from build123d import *

# Parameters (mm, degrees)
F0_W            = 50
F0_H            = 25
F0_R            = 1.6
F0_R_2          = 3.15
F1_DEPTH        = 2.5
F2_R            = 1.5
F3_DEPTH        = 25
F3_COPIES_COUNT = 3
F4_W            = 1.5
F4_H            = 21
F5_DEPTH        = 2


# Not quite as in the source:
# - a pattern or mirror of a feature is missing from the dataset's text; its kind, count and spacing are read off the source's solid


with BuildPart() as f1:
    # F0 (on Top) → F1 (new body)
    with BuildSketch(Plane.XY):
        Rectangle(F0_W, F0_H)
        with Locations((-20, 0)):
            Circle(F0_R, mode=Mode.SUBTRACT)
        Circle(F0_R_2, mode=Mode.SUBTRACT)
        with Locations((20, 0)):
            Circle(F0_R, mode=Mode.SUBTRACT)
    extrude(amount=F1_DEPTH)

    # F2 (on face) → F3 (cut)
    with BuildSketch(Plane.XY.offset(2.5)):
        with Locations((0, 8)):
            Circle(F2_R)
    f3 = extrude(amount=-F3_DEPTH, mode=Mode.SUBTRACT)

    # F3_copies: F3 ×3 about axis
    f3_copies_axis = Axis((0, 0, 0), (0, 0, 1))
    for i in range(1, F3_COPIES_COUNT):
        add(f3.rotate(f3_copies_axis, i * 360 / F3_COPIES_COUNT), mode=Mode.SUBTRACT)

    # F4 (on face) → F5 (join)
    with BuildSketch(Plane.XY.offset(2.5)):
        Polygon((25, 12.5), (-25, 12.5), (-25, 10.5), (-5, 10.5), (-3.5, 10.5), (3.5, 10.5), (5, 10.5), (25, 10.5), align=None)
        with Locations((-4.25, 0)):
            Rectangle(F4_W, F4_H)
        with Locations((4.25, 0)):
            Rectangle(F4_W, F4_H)
        Polygon((-3.5, -10.5), (-5, -10.5), (-25, -10.5), (-25, -12.5), (25, -12.5), (25, -10.5), (5, -10.5), (3.5, -10.5), align=None)
    extrude(amount=F5_DEPTH)


solid = f1.part
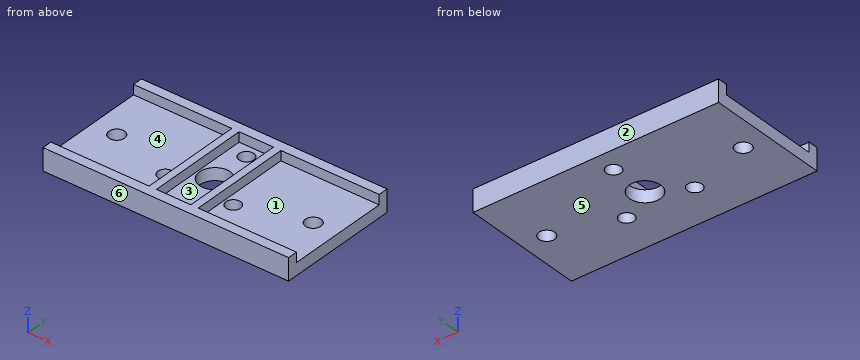
Here's how the part is built. I have some questions about the finished solid (model axes, mm). Face numbers are marked on the shaded views. A direction names the side the tool comes from. Give positions to 0.01 mm unless a question says otherwise; leave off trailing zeros. Loops run counter-clockwise (first coordinate to the right, second up) from the corner with the lowest first, then second, coordinate; pieces in that order, holes last. Notation, with made-up numbers: (-21, 30) -> (-10, 30) arc R31 cw to (-10, 66) -> close; hole circle Ø2 at (28, 68.25). An arc over 180 degrees is marked (long way). Answer as a JSON object with one key per item and string values. Group by question number.
Item 1: Will these pins go through, and if not, where does the flat tip stop? pin 1 (1.9 mm diameter, centred on x = -20, y = 0, fed in from -Z); pin 2 (2 mm diameter, centred on y = 0, z = 4, fed in from -X); pin 3 (2 mm diameter, centred on y = -2, z = 4, fed in from +X); pin 4 (6 mm diameter, centred on x = 8.5, y = -5, fed in from +Z).
Item 2: Imagine slicing it at A-A on y = 0. Write out the boundary of the cut face in (x, z).
Item 3: I need wall thicknesses on L1, parallel to Y at x = 0, z = 1.9; L2, parallel to Y at x = -20, z = 1.35; L3, parallel to X at y = -8, z = 3.45. Which ranges of each line are inside material? Lowest first, please.
Item 4: Imagine slicing it at B-B on x = -20. Write out the boundary of the cut face in (y, z).
Item 5: Imagine slicing it at C-C on x = 0. Write out the boundary of the cut face in (y, z).
Item 6: Imagine slicing it at D-D on y = -4. Write out the boundary of the cut face in (x, z), then the cut area to 3 significant figures.
Item 7: Thinking about a two-plate mould opening in Y: for the marked faces 4, 5 and 6, which applies, pulls with the +Y half, pulls with the -Y half, needs draft (parallel to the pull), parting line crosses it, or undercut?
Item 8: On a 3-axis mill with a long thin cutter (end or side, diameter ignored), from which of +Z, -Z, +X, -X, +Y, -Y can I reach the whole of each face in a straight line? I mean the marked faces 1, 2 and 3. Say none if no direction works.
Answer list:
{
 "1": {"pin 1": "passes through", "pin 2": "stops at x = -5", "pin 3": "stops at x = 5", "pin 4": "stops at z = 2.5"},
 "2": {"outline": "(-25, 0) -> (-21.6, 0) -> (-21.6, 2.5) -> (-25, 2.5) -> close; (-18.4, 0) -> (-3.15, 0) -> (-3.15, 2.5) -> (-3.5, 2.5) -> (-3.5, 4.5) -> (-5, 4.5) -> (-5, 2.5) -> (-18.4, 2.5) -> close; (3.15, 0) -> (18.4, 0) -> (18.4, 2.5) -> (5, 2.5) -> (5, 4.5) -> (3.5, 4.5) -> (3.5, 2.5) -> (3.15, 2.5) -> close; (21.6, 0) -> (25, 0) -> (25, 2.5) -> (21.6, 2.5) -> close"},
 "3": {"L1": "y = -12.5 to -3.15, 3.15 to 6.5, 9.5 to 12.5", "L2": "y = -12.5 to -1.6, 1.6 to 12.5", "L3": "x = -5 to -3.5, 3.5 to 5"},
 "4": {"outline": "(-12.5, 0) -> (-1.6, 0) -> (-1.6, 2.5) -> (-10.5, 2.5) -> (-10.5, 4.5) -> (-12.5, 4.5) -> close; (1.6, 0) -> (12.5, 0) -> (12.5, 4.5) -> (10.5, 4.5) -> (10.5, 2.5) -> (1.6, 2.5) -> close"},
 "5": {"outline": "(-12.5, 0) -> (-3.15, 0) -> (-3.15, 2.5) -> (-10.5, 2.5) -> (-10.5, 4.5) -> (-12.5, 4.5) -> close; (3.15, 0) -> (6.5, 0) -> (6.5, 2.5) -> (3.15, 2.5) -> close; (9.5, 0) -> (12.5, 0) -> (12.5, 4.5) -> (10.5, 4.5) -> (10.5, 2.5) -> (9.5, 2.5) -> close"},
 "6": {"outline": "(-25, 0) -> (-8.43, 0) -> (-8.43, 2.5) -> (-25, 2.5) -> close; (-5.43, 0) -> (5.43, 0) -> (5.43, 2.5) -> (5, 2.5) -> (5, 4.5) -> (3.5, 4.5) -> (3.5, 2.5) -> (-3.5, 2.5) -> (-3.5, 4.5) -> (-5, 4.5) -> (-5, 2.5) -> (-5.43, 2.5) -> close; (8.43, 0) -> (25, 0) -> (25, 2.5) -> (8.43, 2.5) -> close", "area": "116 mm2"},
 "7": {"face 4": "undercut", "face 5": "needs draft", "face 6": "pulls with the -Y half"},
 "8": {"face 1": "+Z, +X", "face 2": "+Z, -Z, +X, -X, +Y", "face 3": "+Z"}
}
